The listing builds one solid part. Answer for the finished solid, in the listing's coordinates (mm). A direction names the side the tool comes from. Coordinates: 2 decimals unless noted, no trailing zeros. Loops run counter-clockwise (first coordinate to the right, second up) from the corner with the lowest first, then second, coordinate; pieces in that order, holes last. Notation, with made-up numbers: (33.5, 41) -> (60.5, 41) arc R16 ccw to (60.5, 60) -> close; hole circle Ø3 at (87, 15.5). An arc over 180 degrees is marked (long way). Answer in a Markdown table with one row per item.
```python
from build123d import *

# Parameters (mm, degrees)
BOSS_EXTRUDE1_DEPTH = 4
SKETCH2_R           = 20
SKETCH2_R_2         = 12.5
SKETCH2_R_3         = 15
SKETCH2_R_4         = 7.5
BOSS_EXTRUDE2_DEPTH = 7.5
SKETCH3_R           = 20
SKETCH3_R_2         = 12.5
BOSS_EXTRUDE3_DEPTH = 15


with BuildPart() as part:
    # Sketch1 → Boss-Extrude1 (new, symmetric)
    with BuildSketch(Plane.XY):
        with BuildLine():
            Line((59.81488788, 13.727342811), (-199.220649297, 19.976731751))
            ThreePointArc((-199.220649297, 19.976731751), (-185.706002057, 13.796933419), (-180.18511212, 0))
            ThreePointArc((-180.18511212, 0), (-185.84170962, -13.937962718), (-199.611792592, -19.991780929))
            Line((-199.611792592, -19.991780929), (59.81488788, -16.272657189))
            ThreePointArc((59.81488788, -16.272657189), (44.81488788, -1.272657189), (59.81488788, 13.727342811))
        make_face()
    extrude(amount=BOSS_EXTRUDE1_DEPTH, both=True)

    # Sketch2 → Boss-Extrude2 (add, symmetric)
    # profile 1 of 2: a face of its own
    with BuildSketch(Plane.XY):
        with Locations((-200.18511212, 0)):
            Circle(SKETCH2_R)
        with Locations((-200.18511212, 0)):
            Circle(SKETCH2_R_2, mode=Mode.SUBTRACT)
    # profile 2 of 2: a face of its own
    with BuildSketch(Plane.XY):
        with Locations((59.81488788, -1.272657189)):
            Circle(SKETCH2_R_3)
        with Locations((59.81488788, -1.272657189)):
            Circle(SKETCH2_R_4, mode=Mode.SUBTRACT)
    extrude(amount=BOSS_EXTRUDE2_DEPTH, both=True)

    # Sketch3 → Boss-Extrude3 (add)
    with BuildSketch(Plane(origin=(0, 0, -7.5), x_dir=(-1, 0, 0), z_dir=(0, 0, -1))):
        with Locations((200.18511212, 0)):
            Circle(SKETCH3_R)
        with Locations((200.18511212, 0)):
            Circle(SKETCH3_R_2, mode=Mode.SUBTRACT)
    extrude(amount=BOSS_EXTRUDE3_DEPTH)


solid = part.part
```
Item 1: A cutting plane is placed at B-B, the plane x = -104. Determine the outline of the cut face in (y, z), plus the area to 3 significant figures.
Findings below:
| item | result |
|---|---|
| outline | (-18.62, -4) -> (17.68, -4) -> (17.68, 4) -> (-18.62, 4) -> close |
| area | 290 mm2 |
Item 2: Determine the mould class of faces 3 (the face through (66.97, 0.98, -0.11)), 4 (the face through (74.122, 3.233, 0.105)), 5 (the face through (-191, -9, -22.5)) for opening direction Y: +Y half, -Y half, draft (parallel to the pull), parting line (faces both ways), or undercut.
Findings below:
| item | result |
|---|---|
| face 3 | undercut |
| face 4 | parting line |
| face 5 | draft |
Item 3: A cutting plane is placed at A-A, the plane z = -15.75. Determine the outline of the cut face in (x, y), plus the area to 3 significant figures.
Findings below:
| item | result |
|---|---|
| outline | circle Ø40 at (-200.19, 0); hole circle Ø25 at (-200.19, 0) |
| area | 766 mm2 |
Item 4: A tool of negligible diameter and unlimited length cuts with its end or side. For faces 1 (the face through (63, 6, 7.5)), 2 (the face through (63, 6, -7.5)), from which of +Z, -Z, +X, -X, +Y, -Y can it reach the whole face along a straight path? Write none if from no direction.
Findings below:
| item | result |
|---|---|
| face 1 | +Z, +X, -X, +Y, -Y |
| face 2 | -Z, +X, +Y, -Y |
Item 5: Find the intervals of material crossed by probe 1 along X at (y, z) = (0, -15.25); probe 2 along X at (y, z) = (-10, -4.75); probe 3 along X at (y, z) = (-9.5, 4.75), in increasing order.
Findings below:
| item | result |
|---|---|
| probe 1 | x = -220.19 to -212.69, -187.69 to -180.19 |
| probe 2 | x = -217.51 to -207.69, -192.69 to -182.86, 47.62 to 72.01 |
| probe 3 | x = -217.78 to -208.31, -192.06 to -182.59, 47.27 to 72.36 |
Item 6: Flat-ended cylindrical pins translate along their axes: pin 1 Ø20 at (x, y) = (-15, -6.5) entering from +Z; pin 2 Ø2 at (y, z) = (3, -7.5) entering from +X; pin 3 Ø17 at (x, y) = (59.81, -1.27) entering from +Z; pin 4 Ø2 at (y, z) = (-4, -19) entering from -X. Find the tip coordinate at first contact, or state that the pin passes through.
Findings below:
| item | result |
|---|---|
| pin 1 | stops at z = 4 |
| pin 2 | stops at x = 74.45 |
| pin 3 | stops at z = 7.5 |
| pin 4 | stops at x = -219.96 |
